```python
from build123d import *

# Parameters (mm, degrees)
PAD_DEPTH       = 18.9
SKETCH001_W     = 30
SKETCH001_H     = 7.9
POCKET_DEPTH    = 26.001
POCKET001_DEPTH = 44.239
SKETCH003_R     = 1.75
POCKET002_DEPTH = 33.4954
SKETCH005_R     = 1.5
POCKET004_DEPTH = 35.001
SKETCH007_R     = 1.2954
SKETCH007_W     = 10.4944
SKETCH007_H     = 13.9
POCKET005_DEPTH = 5.9954
SKETCH008_R     = 1.4986
POCKET006_DEPTH = 0.762


with BuildPart() as part:
    # Sketch → Pad (new body)
    with BuildSketch(Plane.YZ):
        Polygon((-2.5, 2.7564), (-2.5, 1.9944), (-5.4972, 1.9944), (-5.4972, 2.3754), (-7.4972, 2.3754), (-7.4972, 1.9944), (-10.4944, 1.9944), (-10.4944, 2.7564), (-12.4944, 2.7564), (-12.4944, -3.238), (0, -3.238), (0, 6), (24, 6), (24, 41), (20, 41), (10, 11), (-2, 11), (-2, 2.7564), align=None)
    extrude(amount=PAD_DEPTH)

    # Sketch001 (on Face17 of Pad) → Pocket (cut, through all)
    with BuildSketch(Plane(origin=(0, -2, 0), x_dir=(0, 0, -1), z_dir=(0, -1, 0))):
        with Locations((-26, 14.95)):
            Rectangle(SKETCH001_W, SKETCH001_H)
    extrude(amount=-POCKET_DEPTH, mode=Mode.SUBTRACT)

    # Sketch002 (on Face18 of Pocket) → Pocket001 (cut, through all)
    with BuildSketch(Plane(origin=(0, 0, 41), x_dir=(0, -1, 0), z_dir=(0, 0, 1))):
        Polygon((-21, 10), (-21, 1), (-21, 0), (-24, 0), (-24, 1), (-24, 10), align=None)
    extrude(amount=-POCKET001_DEPTH, mode=Mode.SUBTRACT)

    # Sketch003 (on Face26 of Pocket001) → Pocket002 (cut, through all)
    with BuildSketch(Plane.ZX.offset(21)):
        with Locations((13.5, 5.5)):
            Circle(SKETCH003_R)
        with Locations((33.5, 5.5)):
            Circle(SKETCH003_R)
    extrude(amount=-POCKET002_DEPTH, mode=Mode.SUBTRACT)

    # Sketch005 → Pocket004 (cut, through all)
    with BuildSketch(Plane.YX.offset(-6)):
        with Locations((2.5, 14.45)):
            Circle(SKETCH005_R)
        with Locations((17.5, 14.45)):
            Circle(SKETCH005_R)
        with Locations((2.5, 4.45)):
            Circle(SKETCH005_R)
    extrude(amount=-POCKET004_DEPTH, mode=Mode.SUBTRACT)

    # Sketch007 (on Face16 of Pocket004) → Pocket005 (cut, through all)
    with BuildSketch(Plane(origin=(0, 0, 2.7564), x_dir=(0, -1, 0), z_dir=(0, 0, 1))):
        with Locations((8.9958, 2.5)):
            Circle(SKETCH007_R)
        with Locations((3.9986, 2.5)):
            Circle(SKETCH007_R)
        with Locations((7.2472, 11.95)):
            Rectangle(SKETCH007_W, SKETCH007_H)
    extrude(amount=-POCKET005_DEPTH, mode=Mode.SUBTRACT)

    # Sketch008 (on Face17 of Pocket005) → Pocket006 (cut)
    with BuildSketch(Plane(origin=(0, 0, 1.9944), x_dir=(0, -1, 0), z_dir=(0, 0, 1))):
        with Locations((8.9958, 2.5)):
            Circle(SKETCH008_R)
        with Locations((3.9986, 2.5)):
            Circle(SKETCH008_R)
    extrude(amount=-POCKET006_DEPTH, mode=Mode.SUBTRACT)


solid = part.part
```
The listing builds one solid part. Answer for the finished solid, in the listing's coordinates (mm). A direction names the side the tool comes from. Give positions to 0.01 mm unless a question says otherwise; leave off trailing zeros. Loops run counter-clockwise (first coordinate to the right, second up) from the corner with the lowest first, then second, coordinate; pieces in that order, holes last. Notation, with made-up numbers: (13.25, 8) - (52.25, 8) arc R29 cw to (52.25, 40) - close; hole circle Ø7 at (62, 39.25). An arc over 180 degrees is marked (long way). Return JSON: item names as keys, results as strings. Group by question number.
1. Find section B-B (z = 33.5). Write down the section's boundary in (x, y).
2. Given pin 1 Ø4 at (x, y) = (2.5, -9) entering from +Z; pin 2 Ø6 at (y, z) = (3, 5) entering from +X; pin 3 Ø3.5 at (x, y) = (14.45, 2.5) entering from +Z; pin 4 Ø7 at (x, z) = (13.5, 5) entering from -Y, each flat-ended and moving along its own axis, determine where each tip first touches the part or whether it passes through.
3. Which of the six approach directions +Z, -Z, +X, -X, +Y, -Y give full straight-line access (tool end or side, diameter ignored) to faces 4 (the flat face through (9, 12, 6)), 5 (the flat face through (10, 23, 24)), 6 (the flat face through (11, 8, 11)), 7 (the flat face through (0.7, -4, 1.994))?
4. Find section D-D (z = 8.5). Write down the section's boundary in (x, y), then the cut area to 3 significant figures.
5. Find section C-C (y = 2.5). Write down the section's boundary in (x, z).
6. Find section A-A (x = 14.45). Write down the section's boundary in (y, z), then the cut area to 3 significant figures.
7. Determine the mould class of faces 1 (the flat face through (4.3, -9, 1.994)), 2 (the flat face through (5, 15, 26)), 3 (the flat face through (2, -11, 2.756)) for opening direction Y: pulls with the +Y half, pulls with the -Y half, needs draft (parallel to the pull), parting line crosses it, or undercut.
8. Straight lines are drawn through the part: line 1 (Y direction, x = 2.5, z = 1.6); line 2 (X direction, y = 17.5, z = 8.95); line 3 (Z direction, x = 18, y = 10). For each, find the intervals that lie inside material, in ascending order. Write a range as [from, to].
Verdict:
{
 "1": {"outline": "(0, 17.5) - (3.75, 17.5) - (3.75, 21) - (0, 21) - close; (7.25, 17.5) - (11, 17.5) - (11, 24) - (10, 24) - (10, 21) - (7.25, 21) - close"},
 "2": {"pin 1": "stops at z = 2.76", "pin 2": "stops at x = 18.9", "pin 3": "stops at z = 11", "pin 4": "stops at y = -2"},
 "3": {"face 4": "-Z, +X, -X, +Y", "face 5": "+Z, -Z, -X, +Y", "face 6": "+Z, +X, -Y", "face 7": "+Z, +X, -X"},
 "4": {"outline": "(0, -2) - (18.9, -2) - (18.9, 24) - (10, 24) - (10, 21) - (0, 21) - close; hole circle Ø3 at (4.45, 2.5); hole circle Ø3 at (14.45, 2.5); hole circle Ø3 at (14.45, 17.5)", "area": "440 mm^2"},
 "5": {"outline": "(0, 6) - (2.95, 6) - (2.95, 11) - (0, 11) - close; (5.95, 6) - (12.95, 6) - (12.95, 11) - (5.95, 11) - close; (15.95, 6) - (18.9, 6) - (18.9, 11) - (15.95, 11) - close"},
 "6": {"outline": "(-2, -3.24) - (0, -3.24) - (0, 6) - (1, 6) - (1, 11) - (-2, 11) - close; (4, 6) - (16, 6) - (16, 11) - (4, 11) - close; (19, 6) - (24, 6) - (24, 11) - (19, 11) - close", "area": "118 mm^2"},
 "7": {"face 1": "undercut", "face 2": "pulls with the -Y half", "face 3": "needs draft"},
 "8": {"line 1": "y = [-12.49, -10.49], [-7.5, -5.5], [-2.5, 0]", "line 2": "x = [0, 12.95], [15.95, 18.9]", "line 3": "z = [6, 11]"}
}
